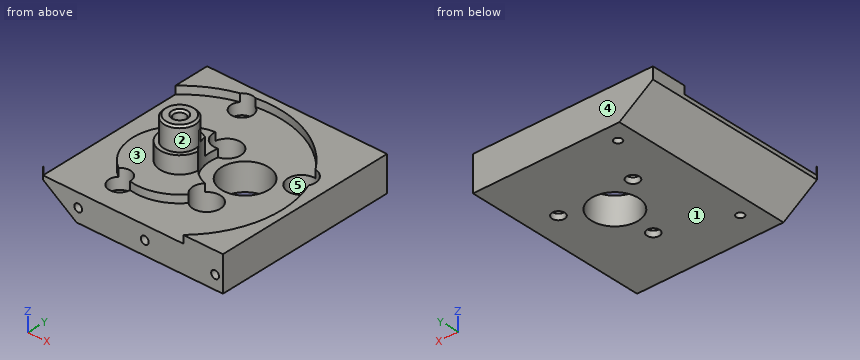
```python
from build123d import *

# Parameters (mm, degrees)
SKETCH_1_W                  = 52
SKETCH_1_H                  = 47
EXTRUDE_336_DEPTH           = 9
SKETCH_2_R                  = 26.1
SKETCH_2_R_2                = 12
CUT_EXTRUDE_544_DEPTH       = 2
SKETCH_3_R                  = 5
EXTRUDE_1_DEPTH             = 4.4
SKETCH_4_R                  = 4
EXTRUDE_2_DEPTH             = 6
SKETCH_5_R                  = 1.5
CUT_EXTRUDE_852_DEPTH       = 10.1
CHAMFER_1_SIZE              = 0.5
CUT_EXTRUDE_1174_DEPTH      = 72.181177287
CUT_EXTRUDE_1174_DEPTH_BACK = 72.181177287
SKETCH_6_R                  = 6
CUT_EXTRUDE_1461_DEPTH      = 72.181177287
CUT_EXTRUDE_1461_DEPTH_BACK = 72.181177287
SKETCH_7_R                  = 1.6
CUT_EXTRUDE_START           = -5.5
SKETCH_8_R                  = 3.5
CUT_EXTRUDE_1708_DEPTH      = 77.681177287
PATTERN_CIRCULAR_1_COUNT    = 3
SKETCH_9_R                  = 1
CUT_EXTRUDE_2077_DEPTH      = 72.181177287
CUT_EXTRUDE_2390_DEPTH      = 72.181177287
CUT_EXTRUDE_2390_DEPTH_BACK = 3
SKETCH_10_R                 = 2.75
SKETCH_11_R                 = 1
CUT_EXTRUDE_9_DEPTH         = 7.5
CUT_EXTRUDE_1_DEPTH         = 73.72798636
CUT_EXTRUDE_2_DEPTH         = 73.72798636
SKETCH_14_R                 = 9
CUT_EXTRUDE_10_DEPTH        = 10


with BuildPart() as part:
    # 草图1 → Extrude 336 (new body)
    with BuildSketch(Plane.XY):
        with Locations((26, 23.5)):
            Rectangle(SKETCH_1_W, SKETCH_1_H)
    extrude(amount=EXTRUDE_336_DEPTH)

    # 草图2 → Cut-Extrude 544 (cut)
    with BuildSketch(Plane.XY.offset(9)):
        with Locations((24, 19)):
            Circle(SKETCH_2_R)
        with Locations((24, 19)):
            Circle(SKETCH_2_R_2, mode=Mode.SUBTRACT)
    extrude(amount=-CUT_EXTRUDE_544_DEPTH, mode=Mode.SUBTRACT)

    # 草图3 → 轮子连接1 (add)
    with BuildSketch(Plane.XY.offset(9)):
        with Locations((24, 19)):
            Circle(SKETCH_3_R)
    extrude(amount=EXTRUDE_1_DEPTH)

    # 草图4 → 轮子连接2 (add)
    with BuildSketch(Plane.XY.offset(13.4)):
        with Locations((24, 19)):
            Circle(SKETCH_4_R)
    extrude(amount=EXTRUDE_2_DEPTH)

    # 草图5 → Cut-Extrude 852 (cut)
    with BuildSketch(Plane.XY.offset(19.4)):
        with Locations((24, 19)):
            Circle(SKETCH_5_R)
    extrude(amount=-CUT_EXTRUDE_852_DEPTH, mode=Mode.SUBTRACT)

    # 倒角1
    chamfer_1_edges = [part.edges().sort_by_distance(p)[0] for p in [
        (20, 19, 19.4),
        (22.5, 19, 19.4),
    ]]
    chamfer(chamfer_1_edges, length=CHAMFER_1_SIZE)

    # 草图6 → Cut-Extrude 1174 (cut, two sides: drawn at the far end of the back side and taken through both)
    with BuildSketch(Plane.XY.offset(7).offset(-CUT_EXTRUDE_1174_DEPTH_BACK)):
        with Locations((35.5, 24.844655678)):
            Circle(SKETCH_6_R)
    extrude(amount=CUT_EXTRUDE_1174_DEPTH + CUT_EXTRUDE_1174_DEPTH_BACK, mode=Mode.SUBTRACT)

    # 草图7 → Cut-Extrude 1461 (cut, two sides: drawn at the far end of the back side and taken through both)
    with BuildSketch(Plane.XY.offset(7).offset(-CUT_EXTRUDE_1461_DEPTH_BACK)):
        with Locations((25.973720558, 30.344655678)):
            Circle(SKETCH_7_R)
        with Locations((45.026279442, 30.344655678)):
            Circle(SKETCH_7_R)
        with Locations((35.5, 13.844655678)):
            Circle(SKETCH_7_R)
    extrude(amount=CUT_EXTRUDE_1461_DEPTH + CUT_EXTRUDE_1461_DEPTH_BACK, mode=Mode.SUBTRACT)

    # 草图8 → Cut-Extrude 1708 (cut)
    with BuildSketch(Plane.XY.offset(7).offset(CUT_EXTRUDE_START)):
        with Locations(Location((45.026279442, 30.344655678, 0), (0, 0, 82.411277971))):
            Circle(SKETCH_8_R)
    cut_extrude_1708 = extrude(amount=CUT_EXTRUDE_1708_DEPTH, mode=Mode.SUBTRACT)

    # 阵列(圆周)1: Cut-Extrude 1708 ×3 about axis
    pattern_circular_1_axis = Axis((35.5, 24.844655678, 0), (0, 0, 1))
    for i in range(1, PATTERN_CIRCULAR_1_COUNT):
        add(cut_extrude_1708.rotate(pattern_circular_1_axis, i * 360 / PATTERN_CIRCULAR_1_COUNT), mode=Mode.SUBTRACT)

    # 草图9 → Cut-Extrude 2077 (cut, through all)
    with BuildSketch(Plane.XY.offset(7)):
        with Locations((19.075932294, 42.344655678)):
            Circle(SKETCH_9_R)
        with Locations((19.075932294, 7.344655678)):
            Circle(SKETCH_9_R)
    extrude(amount=-CUT_EXTRUDE_2077_DEPTH, mode=Mode.SUBTRACT)

    # 草图10 → Cut-Extrude 2390 (cut, two sides: drawn at the far end of the back side and taken through both)
    with BuildSketch(Plane.XY.offset(7).offset(-CUT_EXTRUDE_2390_DEPTH_BACK)):
        with Locations(Location((19.075932294, 42.344655678, 0), (0, 0, 139.177975249))):
            Circle(SKETCH_10_R)
        with Locations(Location((19.075932294, 7.344655678, 0), (0, 0, 137.224544141))):
            Circle(SKETCH_10_R)
    extrude(amount=CUT_EXTRUDE_2390_DEPTH + CUT_EXTRUDE_2390_DEPTH_BACK, mode=Mode.SUBTRACT)

    # 草图11 → 切除-拉伸9 (cut)
    with BuildSketch(Plane.XZ):
        with Locations(Location((15, 3.5, 0), (0, 0, 270))):
            Circle(SKETCH_11_R)
        with Locations(Location((50, 3.5, 0), (0, 0, 270))):
            Circle(SKETCH_11_R)
        with Locations(Location((32, 3.5, 0), (0, 0, 270))):
            Circle(SKETCH_11_R)
    extrude(amount=-CUT_EXTRUDE_9_DEPTH, mode=Mode.SUBTRACT)

    # 草图12 → 修改外形1 (cut, through all)
    with BuildSketch(Plane.XZ):
        Polygon((0, 8), (11.425184054, 0), (0, 0), align=None)
    extrude(amount=-CUT_EXTRUDE_1_DEPTH, mode=Mode.SUBTRACT)

    # 草图13 → 修改外形2 (cut, through all)
    with BuildSketch(Plane(origin=(0, 47, 0), x_dir=(1, 0, 0), z_dir=(0, 1, 0))):
        Polygon((0, -9), (6, -9), (6, -6), (14.56888804, 0), (11.425184054, 0), (0, -8), align=None)
    extrude(amount=-CUT_EXTRUDE_2_DEPTH, mode=Mode.SUBTRACT)

    # 草图14 → 切除-拉伸10 (cut)
    with BuildSketch(Plane.XY.offset(7)):
        with Locations((35.5, 24.844655678)):
            Circle(SKETCH_14_R)
    extrude(amount=CUT_EXTRUDE_10_DEPTH, mode=Mode.SUBTRACT)


solid = part.part
```
Design review of the part built by this model. Coordinates are the model's own, in mm. Face numbers are marked on the shaded views. A direction names the side the tool comes from. Round coordinates to 2 decimals unless told otherwise and drop trailing zeros. Write each loop counter-clockwise with the first axis right and the second up, starting at its lowest first coordinate (ties: lowest second). Pieces come first, ordered by that corner, then holes.
Item 1: We need section C-C on y = 28. Write out the cut boundary in (x, z), and give its area (3 significant figures).
Item 2: Clearance check with flat-ended pins moving along their axes: pin 1 Ø6 at (x, y) = (20, 41.5) entering from +Z; pin 2 Ø1.6 at (x, z) = (32, 3.5) entering from -Y; pin 3 Ø6 at (y, z) = (26, 11.5) entering from -X. State where each tip first meets the part, or that it passes through.
Item 3: For the marked faces 1 and 2, list the 3-axis set-ups (+Z, -Z, +X, -X, +Y, -Y) from which the entire face can be reached by the end or side of a thin tool; tool diameter is ignored.
Item 4: We need section A-A on x = 40. Write out the cut boundary in (y, z).
Item 5: We need section D-D on x = 47.5. Write out the cut boundary in (y, z), and give its area (3 significant figures).
Item 6: The part is to be moulded in two halves that separate along Y. For the marked faces 3, 4 and 5, say which applies: +Y half, -Y half, draft (parallel to the pull), parting line (faces both ways), or undercut.
Item 7: For probe 1 along X at (y, z) = (2, 3.5); probe 2 along Y at (x, z) = (38, 5); probe 3 along X at (y, z) = (27.5, 5.5), list the stretches that pass through material, from the lowest coordinate up.
Item 8: We need section B-B on z = 14.75. Write out the cut boundary in (x, y).
Returned:
1. outline: (6, 6) - (14.57, 0) - (30.4, 0) - (30.4, 7) - (28.57, 7) - (28.57, 1.5) - (23.38, 1.5) - (23.38, 9) - (16.06, 9) - (16.06, 7) - (6, 7) - close; (40.6, 0) - (52, 0) - (52, 9) - (48.5, 9) - (48.5, 7) - (47.62, 7) - (47.62, 1.5) - (42.43, 1.5) - (42.43, 7) - (40.6, 7) - close
1. area: 189 mm2
2. pin 1: stops at z = 7
2. pin 2: stops at y = 7.5
2. pin 3: stops at x = 13.25
3. face 1: -Z, +X, -X, +Y, -Y
3. face 2: +Z
4. outline: (0, 0) - (20.88, 0) - (20.88, 7) - (0, 7) - close; (28.81, 0) - (47, 0) - (47, 9) - (39.62, 9) - (39.62, 7) - (28.81, 7) - close
5. outline: (0, 0) - (47, 0) - (47, 9) - (32.82, 9) - (32.82, 1.5) - (27.87, 1.5) - (27.87, 7) - (7.64, 7) - (7.64, 9) - (0, 9) - close
5. area: 345 mm2
6. face 3: draft
6. face 4: +Y half
6. face 5: undercut
7. probe 1: x = 9.57 to 14, 16 to 31, 33 to 49, 51 to 52
7. probe 2: y = 0 to 11.4, 16.29 to 19.39, 30.3 to 47
7. probe 3: x = 6.71 to 23.93, 28.01 to 30.12, 40.88 to 42.99, 47.07 to 52
8. outline: (27.17, 21.44) arc R4 ccw (long way) to (27.84, 20.12) arc R9 cw to start; hole circle Ø3 at (24, 19)
